Check sheet for the modelled part. Datum: model origin and axes. Units: mm. A direction names the side the tool comes from. Round coordinates to 2 decimals unless told otherwise and drop trailing zeros. Write each loop counter-clockwise with the first axis right and the second up, starting at its lowest first coordinate (ties: lowest second). Pieces come first, ordered by that corner, then holes.
Item 1: Material ranges on line 1 along X through (y, z) = (10.5, 13); line 2 along X through (y, z) = (5, 8.5); line 3 along X through (y, z) = (9.25, 9.5), recorded low to high.
Item 2: Section check A-A, the plane z = 11.75. Record the cut outline in (x, y) (1 decimal).
Item 3: Set-up check for faces 1 (the flat face through (-10.381, 7, 9)), 2 (the flat face through (6, 14.288, 10)), 3 (the flat face through (-13, 7, 14.288)): record each of +Z, -Z, +X, -X, +Y, -Y from which the full face is reachable in a straight line by a thin tool's end or side.
Item 4: Release check for a two-part mould opening along Z. For faces 4 (the flat face through (0, 14, 19.05)), 5 (the flat face through (-13, 7, 4.762)), 6 (the cylindrical face through (5.43, 11.87, 5.65)), 7 (the cylindrical face through (-1.464, 20.585, 9.392)) record: pulls with the +Z half, pulls with the -Z half, needs draft (parallel to the pull), parting line crosses it, or undercut.
Item 5: Depth check by flat-ended pin: pin 1 (1.4 mm diameter, centred on y = 7.5, z = 11, fed in from +X); pin 2 (2.5 mm diameter, centred on x = 7.5, z = 9.5, fed in from -Y); pin 3 (10 mm diameter, centred on x = 6.5, z = 11.5, fed in from -Y) (3 decimals). Enter the tip coordinate at first touch or a pass-through.
Item 6: Section check C-C, the plane y = 3. Record the cut outline in (x, z).
from build123d import *

# Parameters (mm, degrees)
F1_DEPTH = 19.05
F2_W     = 4.7625
F2_H     = 4.7625
F3_DEPTH = 25.4
F4_R     = 2.38125
F5_DEPTH = 14.2885
F6_R     = 3.96875
F7_DEPTH = 4.7625


with BuildPart() as f1:
    # F0 (on Top) → F1 (new body)
    with BuildSketch(Plane.XY):
        with BuildLine():
            Line((-10.381285, 9.525), (18.307943, 9.525))
            ThreePointArc((18.307943, 9.525), (-1.803848, 20.558515), (-19.68692, 6.19125))
            ThreePointArc((-19.68692, 6.19125), (-15.866531, 0.055161), (-10.381285, 4.7625))
            Line((-10.381285, 4.7625), (-10.381285, 9.525))
        make_face()
    extrude(amount=F1_DEPTH)

    # F2 (on face) → F3 (cut)
    with BuildSketch(Plane.YZ.offset(-10.381285)):
        with Locations((7.14375, 16.66875)):
            Rectangle(F2_W, F2_H)
        with Locations((2.38125, 16.66875)):
            Rectangle(F2_W, F2_H)
        with Locations((7.14375, 2.38125)):
            Rectangle(F2_W, F2_H)
        with Locations((2.38125, 2.38125)):
            Rectangle(F2_W, F2_H)
    extrude(amount=-F3_DEPTH, mode=Mode.SUBTRACT)

    # F4 (on face) → F5 (cut, through all)
    with BuildSketch(Plane.XY.offset(14.2875)):
        with Locations((-15.143785, 4.7625)):
            Circle(F4_R)
    extrude(amount=-F5_DEPTH, mode=Mode.SUBTRACT)

    # F6 (on face) → F7 (cut)
    with BuildSketch(Plane.XZ.offset(-9.525)):
        with Locations((6.287465, 9.525)):
            Circle(F6_R)
    extrude(amount=-F7_DEPTH, mode=Mode.SUBTRACT)


solid = f1.part
Values found:
1. line 1: x = -17.77 to 4.37, 8.2 to 17.77
1. line 2: x = -19.9 to -17.51, -12.77 to -10.38
1. line 3: x = -18.45 to -10.38
2. outline: (-19.7, 6.2) arc R4.8 ccw (long way) to (-10.4, 4.8) - (-10.4, 9.5) - (3, 9.5) - (3, 14.3) - (9.6, 14.3) - (9.6, 9.5) - (18.3, 9.5) arc R20.6 ccw to start; hole circle Ø4.8 at (-15.1, 4.8)
3. face 1: +Z, -Z, +X, -Y
3. face 2: -Y
3. face 3: +Z, +X, -X, -Y
4. face 4: pulls with the +Z half
4. face 5: pulls with the -Z half
4. face 6: undercut
4. face 7: needs draft
5. pin 1: stops at x = -10.38
5. pin 2: stops at y = 14.29
5. pin 3: stops at y = 9.525
6. outline: (-19.57, 4.76) - (-16.75, 4.76) - (-16.75, 14.29) - (-19.57, 14.29) - close; (-13.54, 4.76) - (-10.72, 4.76) - (-10.72, 14.29) - (-13.54, 14.29) - close
